from build123d import *

# Parameters (mm, degrees)
CYLINDER001_R       = 1.75
CYLINDER001_DEPTH   = 10
CYLINDER002_R       = 1.75
CYLINDER002_DEPTH   = 10
CYLINDER003_R       = 1.75
CYLINDER003_DEPTH   = 10
CYLINDER_R          = 1.75
CYLINDER_DEPTH      = 10
BOX001_W            = 189.5
BOX001_H            = 26.75
BOX001_DEPTH        = 70
BOX_W               = 208
BOX_H               = 89.3
BOX_DEPTH           = 2
FILLET_R            = 2.5
CUT_PLACEMENT_ANGLE = 90


with BuildPart() as cylinder001:
    # Cylinder001 → Cylinder001 (new body)
    with BuildSketch(Plane(origin=(5.4, 82.6, 0), x_dir=(1, 0, 0), z_dir=(0, 0, 1))):
        Circle(CYLINDER001_R)
    extrude(amount=CYLINDER001_DEPTH)


with BuildPart() as cylinder002:
    # Cylinder002 → Cylinder002 (new body)
    with BuildSketch(Plane(origin=(203, 82.6, 0), x_dir=(1, 0, 0), z_dir=(0, 0, 1))):
        Circle(CYLINDER002_R)
    extrude(amount=CYLINDER002_DEPTH)


with BuildPart() as cylinder003:
    # Cylinder003 → Cylinder003 (new body)
    with BuildSketch(Plane(origin=(203, 6.4, 0), x_dir=(1, 0, 0), z_dir=(0, 0, 1))):
        Circle(CYLINDER003_R)
    extrude(amount=CYLINDER003_DEPTH)


with BuildPart() as base_hole:
    # Cylinder → Cylinder (new body)
    with BuildSketch(Plane(origin=(5.4, 6.4, 0), x_dir=(1, 0, 0), z_dir=(0, 0, 1))):
        Circle(CYLINDER_R)
    extrude(amount=CYLINDER_DEPTH)

    # Fusion: union Cylinder001, Cylinder002, Cylinder003
    add(cylinder001.part)
    add(cylinder002.part)
    add(cylinder003.part)


with BuildPart() as base_hole_1:
    # Fusion placement: moved
    add(base_hole.part.moved(Location((0, 0, -4))))


with BuildPart() as ozone_monitor:
    # Box001 → Box001 (new body)
    with BuildSketch(Plane(origin=(9.5, 62.5, 2), x_dir=(1, 0, 0), z_dir=(0, 0, 1))):
        with Locations((94.75, 13.375)):
            Rectangle(BOX001_W, BOX001_H)
    extrude(amount=BOX001_DEPTH)


with BuildPart() as ozone_module:
    # Box → Box (new body)
    with BuildSketch(Plane.XY):
        with Locations((104, 44.65)):
            Rectangle(BOX_W, BOX_H)
    extrude(amount=BOX_DEPTH)

    # Fillet
    fillet_edges = [ozone_module.edges().sort_by_distance(p)[0] for p in [
        (0, 0, 1),
        (0, 89.3, 1),
        (208, 0, 1),
        (208, 89.3, 1),
    ]]
    fillet(fillet_edges, radius=FILLET_R)

    # Fusion001: union Ozone_monitor
    add(ozone_monitor.part)

    # Cut: cut Base_hole
    add(base_hole_1.part, mode=Mode.SUBTRACT)


with BuildPart() as ozone_module_1:
    # Cut placement: moved
    add(ozone_module.part.moved(Location((-135, 157, 89.2))).rotate(Axis((-135, 157, 89.2), (1, 0, 0)), CUT_PLACEMENT_ANGLE))


solid = ozone_module_1.part
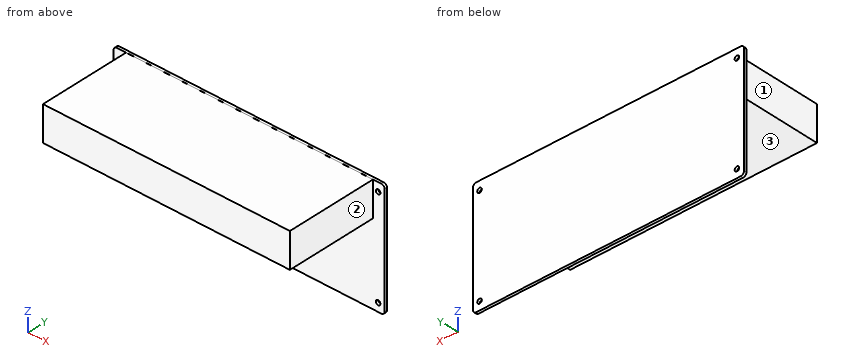
Source: CAD feature listing. Evaluate the final solid. Frame: model axes, mm. Face numbers are marked on the shaded views. A direction names the side the tool comes from. Give positions to 0.01 mm unless a question says otherwise; leave off trailing zeros. Order: outer loops, then holes, each group sorted by start corner. A loop starts at its lowest first (then second) coordinate and runs counter-clockwise, first axis right, second up. Notation, with made-up numbers: (33.25, 83.5) -> (85.25, 83.5) arc R27 cw to (85.25, 118.5) -> close; hole circle Ø4 at (-29, 57). An arc over 180 degrees is marked (long way). Write item = value, one per line.
Q1. Material intervals for line 1 (X direction, y = 155.65, z = 171.8); line 2 (Z direction, x = 68, y = 155.7); line 3 (X direction, y = 156, z = 171), sorted ascending. Write a range as from..to.
Data:
line_1 = -135..-131.35, -127.85..66.25, 69.75..73
line_2 = 89.2..93.85, 97.35..170.05, 173.55..178.5
line_3 = -135..-131.16, -128.04..66.44, 69.56..73
Q2. Cut plane A-A, the plane x = -66.5. Output: boundary loops of the cut face in (y, z).
Data:
outline = (85, 151.7) -> (155, 151.7) -> (155, 89.2) -> (157, 89.2) -> (157, 178.5) -> (155, 178.5) -> (155, 178.45) -> (85, 178.45) -> close
Q3. Pin query (flat end, axial travel): pin 1 (5.5 mm diameter, centred on x = 68, z = 171.8, fed in from -Y); pin 2 (4 mm diameter, centred on x = 13.5, y = 108, fed in from +Z); pin 3 (21 mm diameter, centred on x = -29, y = 133.5, fed in from -Z). Return the tip coordinate at first contact, or that it passes through.
Data:
pin_1 = 155
pin_2 = 178.45
pin_3 = 151.7
Q4. Cut plane C-C, the plane y = 112. Output: boundary loops of the cut face in (x, z).
Data:
outline = (-125.5, 151.7) -> (64, 151.7) -> (64, 178.45) -> (-125.5, 178.45) -> close
Q5. Cut plane B-B, the plane z = 154. Output: boundary loops of the cut face in (x, y), and give its area (3 significant figures).
Data:
outline = (-135, 155) -> (-125.5, 155) -> (-125.5, 85) -> (64, 85) -> (64, 155) -> (73, 155) -> (73, 157) -> (-135, 157) -> close
area = 13,700 mm^2
Q6. Cut plane D-D, the plane z = 123. Output: boundary loops of the cut face in (x, y).
Data:
outline = (-135, 155) -> (73, 155) -> (73, 157) -> (-135, 157) -> close
Q7. Set-up query: the marked faces 1, 2 and 3. Return all of +Z, -Z, +X, -X, +Y, -Y with unobstructed straight access to the full face (end or side cutting, diameter ignored); none if empty.
Data:
face_1 = +Z, -Z, -X, -Y
face_2 = +Z, -Z, +X, -Y
face_3 = -Z, +X, -X, -Y
